Geometry: final body of the model. Coordinates: model frame, mm. A direction names the side the tool comes from. Give positions to 0.01 mm unless a question says otherwise; leave off trailing zeros. Write each loop counter-clockwise with the first axis right and the second up, starting at its lowest first coordinate (ties: lowest second). Pieces come first, ordered by that corner, then holes.
```python
from build123d import *

# Parameters (mm, degrees)
EXTRUDE1_DEPTH = 31.75
FILLET1_R      = 2.54


with BuildPart() as part:
    # Sketch1 → Extrude1 (new body)
    with BuildSketch(Plane.XY):
        Polygon((19.05, 101.6), (19.05, 19.05), (101.6, 19.05), (101.6, 0), (0, 0), (0, 101.6), align=None)
    extrude(amount=EXTRUDE1_DEPTH)

    # Fillet1
    fillet1_edges = [part.edges().sort_by_distance(p)[0] for p in [
        (19.05, 19.05, 15.875),
    ]]
    fillet(fillet1_edges, radius=FILLET1_R)


solid = part.part
```
Item 1: Line query: L1, parallel to Y at x = 33, z = 29. Output: solid intervals per line, ascending.
Found:
L1: y = 0 to 19.05
Item 2: Section B-B, the plane x = 23.5. Return the cut outline in (y, z), plus the area to 3 significant figures.
Found:
outline: (0, 0) - (19.05, 0) - (19.05, 31.75) - (0, 31.75) - close
area: 605 mm2
Item 3: Section A-A, the plane z = 8. Return the cut outline in (x, y), plus the area to 3 significant figures.
Found:
outline: (0, 0) - (101.6, 0) - (101.6, 19.05) - (21.59, 19.05) arc R2.54 cw to (19.05, 21.59) - (19.05, 101.6) - (0, 101.6) - close
area: 3,510 mm2
Item 4: Pin query (flat end, axial travel): pin 1 Ø1.5 at (x, z) = (26, 26.5) entering from +Y; pin 2 Ø8 at (y, z) = (76, 5) entering from +X. Return the tip coordinate at first contact, or that it passes through.
Found:
pin 1: stops at y = 19.05
pin 2: stops at x = 19.05
Item 5: Reachability of faces 1 (the face through (0, 50, 16)), 2 (the face through (61, 19.05, 16)) from +Z, -Z, +X, -X, +Y, -Y: full face, straight path, thin tool, end or side. Return the list, or none.
Found:
face 1: +Z, -Z, -X, +Y, -Y
face 2: +Z, -Z, +X, +Y
